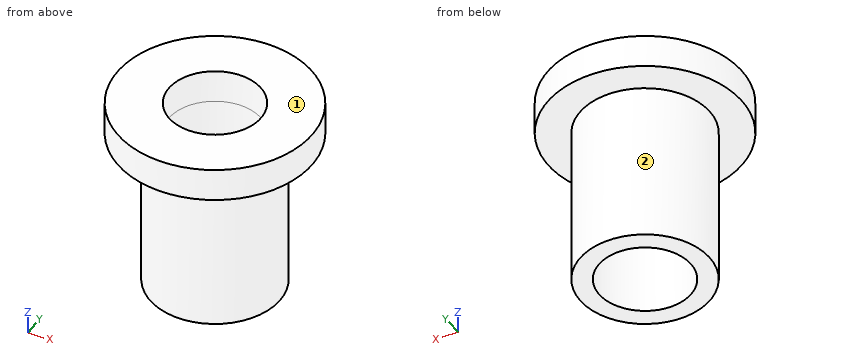
```python
from build123d import *

# Parameters (mm, degrees)
SKETCH_1_R      = 9.5
SKETCH_1_R_2    = 4.5
EXTRUDE_1_DEPTH = 3.25
EXTRUDE_START   = 15.85
SKETCH_2_R      = 6.35
SKETCH_2_R_2    = 4.5
EXTRUDE_2_DEPTH = 15.85


with BuildPart() as part:
    # Эскиз1 → Бобышка-Вытянуть1 (new body)
    with BuildSketch(Plane.XY):
        with Locations(Location((0, 0, 0), (0, 0, 180))):
            Circle(SKETCH_1_R)
        with Locations(Location((0, 0, 0), (0, 0, 180))):
            Circle(SKETCH_1_R_2, mode=Mode.SUBTRACT)
    extrude(amount=EXTRUDE_1_DEPTH)

    # Эскиз2 → Бобышка-Вытянуть2 (add)
    with BuildSketch(Plane(origin=(0, 0, 0), x_dir=(-1, 0, 0), z_dir=(0, 0, -1)).offset(EXTRUDE_START)):
        with Locations(Location((0, 0, 0), (0, 0, 180))):
            Circle(SKETCH_2_R)
        Circle(SKETCH_2_R_2, mode=Mode.SUBTRACT)
    extrude(amount=-EXTRUDE_2_DEPTH)


solid = part.part
```
Part model, mm, in its own coordinate system. Face numbers are marked on the shaded views. A direction names the side the tool comes from. Round coordinates to 2 decimals unless told otherwise and drop trailing zeros. Write each loop counter-clockwise with the first axis right and the second up, starting at its lowest first coordinate (ties: lowest second). Pieces come first, ordered by that corner, then holes. Notation, with made-up numbers: (63.25, 59) -> (98.25, 59) arc R34 ccw to (98.25, 97) -> close; hole circle Ø6 at (48, 45). An arc over 180 degrees is marked (long way). Return JSON: item names as keys, results as strings. Group by question number.
Q1. Which spindle directions (+Z, -Z, +X, -X, +Y, -Y) get a long thin tool onto all of the face, cutting with end or side? Do the marked faces 1 and 2. Say none if no direction does.
Q2. Saw through at D-D on x = 6. Write the cut outline in (y, z).
Q3. Saw through at C-C on z = -6. Write the cut outline in (x, y).
Q4. Saw through at A-A on y = 0. Write the cut outline in (x, z).
Q5. Probe L1, parallel to Y at x = 0, z = -6; L2, parallel to Z at x = -6.75, y = -1; L3, parallel to Y at x = -3, z = -7.25. List the from-to ranges inside material, lowest first. Write a range as [from, to].
Q6. Pin check, flat tips, straight feed: pin 1 (6 mm diameter, centred on x = 5, z = -11, fed in from +Y); pin 2 (1.5 mm diameter, centred on x = 6.5, z = -3.5, fed in from +Y); pin 3 (8 mm diameter, centred on y = -5.5, z = -13.5, fed in from +X); pin 4 (5.5 mm diameter, centred on x = 0, y = 0, fed in from +Z). Stop position of each tip, or through.
Answer:
{
 "1": {"face 1": "+Z, +X, -X, +Y, -Y", "face 2": "-Z"},
 "2": {"outline": "(-7.37, 0) -> (-2.08, 0) -> (-2.08, -15.85) -> (2.08, -15.85) -> (2.08, 0) -> (7.37, 0) -> (7.37, 3.25) -> (-7.37, 3.25) -> close"},
 "3": {"outline": "circle Ø12.7 at (0, 0); hole circle Ø9 at (0, 0)"},
 "4": {"outline": "(-9.5, 0) -> (-6.35, 0) -> (-6.35, -15.85) -> (-4.5, -15.85) -> (-4.5, 3.25) -> (-9.5, 3.25) -> close; (4.5, -15.85) -> (6.35, -15.85) -> (6.35, 0) -> (9.5, 0) -> (9.5, 3.25) -> (4.5, 3.25) -> close"},
 "5": {"L1": "[-6.35, -4.5], [4.5, 6.35]", "L2": "[0, 3.25]", "L3": "[-5.6, -3.35], [3.35, 5.6]"},
 "6": {"pin 1": "y = 6.03", "pin 2": "y = 2.69", "pin 3": "x = 6.17", "pin 4": "through"}
}
